Can you work these out from the model? Positions are in its coordinate system, mm. Give positions to 0.01 mm unless a question says otherwise; leave off trailing zeros. Order: outer loops, then holes, each group sorted by start corner. A loop starts at its lowest first (then second) coordinate and runs counter-clockwise, first axis right, second up. Notation, with made-up numbers: (-31, -16) -> (11, -16) arc R22 cw to (11, -1) -> close; hole circle Ø8 at (8, 37). An arc over 180 degrees is marked (long way). Answer as CSV lines item,"result".
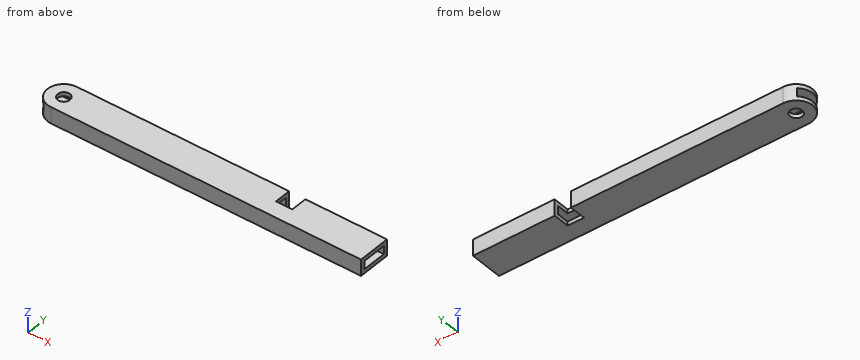
```python
from build123d import *

# Parameters (mm, degrees)
F0_W          = 254
F0_H          = 25.4
F1_DEPTH      = 6.35
F2_R          = 12.69999
F3_R          = 4.7625
F4_DEPTH      = 12.701
F5_W          = 19.05
F5_H          = 6.35
F6_DEPTH      = 127.001
F6_DEPTH_BACK = 127.001
F7_W          = 12.7
F7_H          = 12.7
F8_DEPTH      = 12.701


# Not quite as in the source:
# - a fillet or chamfer is up to 0.001 mm smaller than in the source, because OpenCascade refuses the exact size


with BuildPart() as f1:
    # F0 (on Top) → F1 (new body, symmetric)
    with BuildSketch(Plane.XY):
        Rectangle(F0_W, F0_H)
    extrude(amount=F1_DEPTH, both=True)

    # F2 (radius 12.7 in the source; OpenCascade refuses exactly that, so slightly less here)
    f2_edges = [f1.edges().sort_by_distance(p)[0] for p in [
        (-127, 12.7, 0),
        (-127, -12.7, 0),
    ]]
    fillet(f2_edges, radius=F2_R)

    # F3 (on face) → F4 (cut, through all)
    with BuildSketch(Plane.XY.offset(6.35)):
        with Locations((-114.3, 0)):
            Circle(F3_R)
    extrude(amount=-F4_DEPTH, mode=Mode.SUBTRACT)

    # F5 (on Right) → F6 (cut, two sides)
    with BuildSketch(Plane.YZ) as f6_sk:
        Rectangle(F5_W, F5_H)
    extrude(amount=-F6_DEPTH, mode=Mode.SUBTRACT)
    extrude(f6_sk.sketch, amount=F6_DEPTH_BACK, mode=Mode.SUBTRACT)

    # F7 (on face) → F8 (cut, through all)
    with BuildSketch(Plane.XY.offset(6.35)):
        with Locations((57.15, 6.35)):
            Rectangle(F7_W, F7_H)
    extrude(amount=-F8_DEPTH, mode=Mode.SUBTRACT)


solid = f1.part
```
Item 1: For pin 1 (3 mm diameter, centred on y = 4.5, z = -1, fed in from +X); pin 2 (1.5 mm diameter, centred on y = 4.5, z = -3, fed in from -X); pin 3 (1 mm diameter, centred on x = 58.5, z = 4.5, fed in from +Y), each with a flat end and sliding along its axis, tell me the tip position at first contact or that it passes through.
Numbers:
pin 1,"passes through"
pin 2,"stops at x = -126.43"
pin 3,"stops at y = 0"
Item 2: Please list where these lines run through material, in increasing order: line 1 along Z through (x, y) = (66, -2.5) (3 decimals); line 2 along Y through (x, z) = (-21, -0.5) (3 decimals); line 3 along Y through (x, z) = (-114.3, -5.6).
Numbers:
line 1,"z = -6.35 to -3.175, 3.175 to 6.35"
line 2,"y = -12.7 to -9.525, 9.525 to 12.7"
line 3,"y = -12.7 to -4.76, 4.76 to 12.7"
Item 3: Imagine slicing it at C-C, the plane y = -7. Please give me the cut outline in (x, z) (3 decimals).
Numbers:
outline,"(-124.897, -6.35) -> (127, -6.35) -> (127, -3.175) -> (-124.897, -3.175) -> close; (-124.897, 3.175) -> (127, 3.175) -> (127, 6.35) -> (-124.897, 6.35) -> close"
Item 4: Imagine slicing it at B-B, the plane z = -0.5. Please give me the cut outline in (x, y) (3 decimals).
Numbers:
outline,"(-122.7, -9.525) arc R12.7 ccw to (-114.3, -12.7) -> (127, -12.7) -> (127, -9.525) -> close; (-122.7, 9.525) -> (50.8, 9.525) -> (50.8, 12.7) -> (-114.3, 12.7) arc R12.7 ccw to start; (63.5, 9.525) -> (127, 9.525) -> (127, 12.7) -> (63.5, 12.7) -> close"
Item 5: Imagine slicing it at A-A, the plane x = 38.5. Please give me the cut outline in (y, z) (3 decimals), then the cut area to 3 significant figures.
Numbers:
outline,"(-12.7, -6.35) -> (12.7, -6.35) -> (12.7, 6.35) -> (-12.7, 6.35) -> close; hole (-9.525, -3.175) -> (9.525, -3.175) -> (9.525, 3.175) -> (-9.525, 3.175) -> close"
area,"202 mm²"
